Autodesk Inventor part; units mm, degrees
ref_plane "YZ Plane" through (0, 0, 0) normal (1, 0, 0) x (0, 1, 0)
ref_plane "XZ Plane" through (0, 0, 0) normal (0, 1, 0) x (-1, 0, 0)
ref_plane "XY Plane" through (0, 0, 0) normal (0, 0, 1) x (1, 0, 0)
sketch "Esquisse1" plane through (0, 0, 0) normal (0, 1, 0) x (-1, 0, 0)
  line L0 (-75, 75) -> (75, 75)
  line L1 (75, 75) -> (75, -75)
  line L2 (75, -75) -> (-75, -75)
  line L3 (-75, -75) -> (-75, 75)
  point P0 (0, 0)
  dimension "d0" = 150
  dimension "d1" = 75
  dimension "d2" = 150
  dimension "d3" = 75
extrude "Extrusion1" add sketch "Esquisse1" along normal blind 10
sketch "Esquisse2" plane through (0, 10, 0) normal (0, 1, 0) x (1, 0, 0)
  circle A0 centre (0, 0) radius 5
  dimension "d6" = 10
extrude "Extrusion2" cut sketch "Esquisse2" against normal through all
sketch "Esquisse4" plane through (0, 0, 0) normal (0, -1, 0) x (1, 0, 0)
  circle A0 centre (-65, 65) radius 2
  circle A1 centre (65, 65) radius 2
  circle A2 centre (65, -65) radius 2
  circle A3 centre (-65, -65) radius 2
  line L0 (-75, 75) -> (-75, -75)
  line L1 (75, -75) -> (75, 75)
  line L2 (75, 75) -> (-75, 75)
  line L3 (-75, -75) -> (75, -75)
  point P0 (0, 0)
  dimension "d12" = 4
  dimension "d13" = 4
  dimension "d14" = 4
  dimension "d15" = 4
  dimension "d16" = 10
  dimension "d17" = 10
  dimension "d18" = 10
  dimension "d19" = 10
  dimension "d20" = 10
  dimension "d21" = 10
  dimension "d22" = 10
  dimension "d23" = 10
extrude "Extrusion4" cut sketch "Esquisse4" against normal blind 1 contours A0 | A1 | A2 | A3
equation "\"d13\" = d12"
equation "\"d14\" = d12"
equation "\"d15\" = d12"
equation "\"d17\" = d16"
equation "\"d18\" = d16"
equation "\"d19\" = d16"
equation "\"d20\" = d16"
equation "\"d21\" = d16"
equation "\"d22\" = d16"
equation "\"d23\" = d16"
equation "\"dd0\" = 16"
equation "\"dd1\" = 28"
properties part number "Base" material "PVC, non plastifié"
CAD build for the part. Positions are in the model's coordinates, mm. A direction names the side the tool comes from. Round coordinates to 2 decimals unless told otherwise and drop trailing zeros. Write each loop counter-clockwise with the first axis right and the second up, starting at its lowest first coordinate (ties: lowest second). Pieces come first, ordered by that corner, then holes.
(1) Probe line 1 along Z through (x, y) = (65, 0.35); line 2 along Z through (x, y) = (0, 5.5); line 3 along X through (y, z) = (5, 3). List the from-to ranges inside material, lowest first.
(2) Slice it at B-B, the plane z = 0. Write the cut outline in (x, y).
(3) Mould opens along X. For faces 3 (the face through (-1.08, 5.07, 4.88)), 4 (the face through (-75, 5, 1)), 5 (the face through (1, 10, 18)) say: pulls with the +X half, pulls with the -X half, needs draft (parallel to the pull), parting line crosses it, or undercut.
(4) 3-axis set-ups, long thin cutter, end or side, ignore diameter. For faces 1 (the face through (75, 5, -1)), 2 (the face through (-65, 1, -65)): which of +Z, -Z, +X, -X, +Y, -Y reach the whole face in a straight line?
(5) Drop flat-ended pins along their axis: P1, Ø3, axis at x = 65, z = -65, coming from the -Y side; P2, Ø8, axis at x = 0, z = 0, coming from the -Y side. Give the stop position or say it passes through.
(6) Slice it at A-A, the plane x = 0. Write the cut outline in (y, z), and give its area (3 significant figures).
From the geometry:
1. line 1: z = -75 to -67, -63 to 63, 67 to 75
1. line 2: z = -75 to -5, 5 to 75
1. line 3: x = -75 to -4, 4 to 75
2. outline: (-75, 0) - (-5, 0) - (-5, 10) - (-75, 10) - close; (5, 0) - (75, 0) - (75, 10) - (5, 10) - close
3. face 3: undercut
3. face 4: pulls with the -X half
3. face 5: needs draft
4. face 1: +Z, -Z, +X, +Y, -Y
4. face 2: -Y
5. P1: stops at y = 1
5. P2: passes through
6. outline: (0, -75) - (10, -75) - (10, -5) - (0, -5) - close; (0, 5) - (10, 5) - (10, 75) - (0, 75) - close
6. area: 1,400 mm2
